Geometry check sheet. Reference: the model listing, model coordinates, mm. Coordinates: 2 decimals unless noted, no trailing zeros. Write each loop counter-clockwise with the first axis right and the second up, starting at its lowest first coordinate (ties: lowest second). Pieces come first, ordered by that corner, then holes. Notation, with made-up numbers: (40.5, 37) -> (63.5, 37) arc R27 cw to (63.5, 59) -> close; hole circle Ø3 at (62, 18). An arc over 180 degrees is marked (long way). Answer in a Markdown table with one row per item. Add a question column.
Q1. Section check A-A, the plane x = 38.5. Record the boundary of the cut face in (y, z).
Q2. Section check B-B, the plane z = 0.7. Record the boundary of the cut face in (x, y), and give its area (3 significant figures).
Q3. Gauge pin test, flat end, axial feed: P1, Ø2, axis at x = 34.5, y = -20, coming from the -Z side. Record the tip position at first contact, or that the pin passes through.
Q4. Thickness scan on line 1 (Y direction, x = 40.9, z = 0.9); line 2 (Y direction, x = 27, z = 1.45); line 3 (X direction, y = 9.5, z = 1.4). Record the ranges inside material, lowest first.
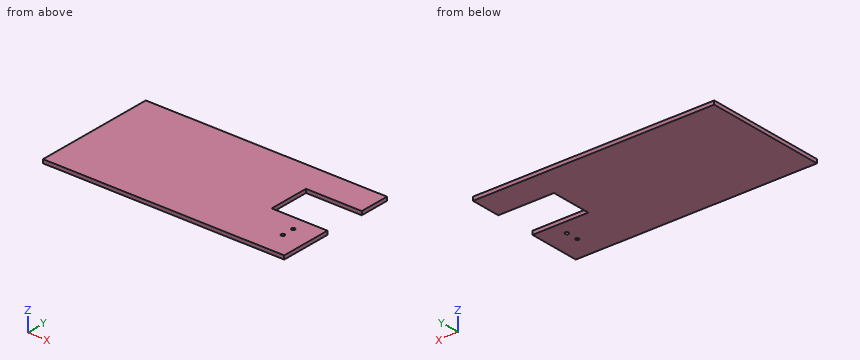
```python
from build123d import *

# Parameters (mm, degrees)
F0_W     = 100
F0_H     = 51
F1_DEPTH = 1.52
F2_W     = 23.136646
F2_H     = 17
F2_R     = 0.75
F3_DEPTH = 25


with BuildPart() as f1:
    # F0 (on Top) → F1 (new body)
    with BuildSketch(Plane.XY):
        Rectangle(F0_W, F0_H)
    extrude(amount=F1_DEPTH)

    # F2 (on face) → F3 (cut)
    with BuildSketch(Plane.XY.offset(1.52)):
        with Locations((38.431677, 4.47)):
            Rectangle(F2_W, F2_H)
        with Locations((40.9, -10.2)):
            Circle(F2_R)
        with Locations((40.9, -15.28)):
            Circle(F2_R)
    extrude(amount=-F3_DEPTH, mode=Mode.SUBTRACT)


solid = f1.part
```
Calculated:
| question | item | result |
|---|---|---|
| 1 | outline | (-25.5, 0) -> (-4.03, 0) -> (-4.03, 1.52) -> (-25.5, 1.52) -> close; (12.97, 0) -> (25.5, 0) -> (25.5, 1.52) -> (12.97, 1.52) -> close |
| 2 | outline | (-50, -25.5) -> (50, -25.5) -> (50, -4.03) -> (26.86, -4.03) -> (26.86, 12.97) -> (50, 12.97) -> (50, 25.5) -> (-50, 25.5) -> close; hole circle Ø1.5 at (40.9, -15.28); hole circle Ø1.5 at (40.9, -10.2) |
| 2 | area | 4,700 mm² |
| 3 | P1 | stops at z = 0 |
| 4 | line 1 | y = -25.5 to -16.03, -14.53 to -10.95, -9.45 to -4.03, 12.97 to 25.5 |
| 4 | line 2 | y = -25.5 to -4.03, 12.97 to 25.5 |
| 4 | line 3 | x = -50 to 26.86 |
